The listing builds one solid part. Answer for the finished solid, in the listing's coordinates (mm). Give positions to 0.01 mm unless a question says otherwise; leave off trailing zeros. Loops run counter-clockwise (first coordinate to the right, second up) from the corner with the lowest first, then second, coordinate; pieces in that order, holes last. Notation, with made-up numbers: M 24,35.5 L 29,35.5 A32 ccw 29,68.5 Z; hole C -24,45.5 d10. An arc over 180 degrees is marked long. Use one line per item in the form item = value. Start each with the question number.
1. The part is cut by section A-A (z = 0). Write down the section's boundary in (x, y) (3 decimals), and give its area (3 significant figures).
2. The part is cut by section D-D (z = -21.5). Write down the section's boundary in (x, y), and give its area (3 significant figures).
3. The part is cut by section B-B (x = 0). Write down the section's boundary in (y, z) (3 decimals), and give its area (3 significant figures).
4. The part is cut by section C-C (y = 42). Give the number of separate pieces and of enclosed holes in the cut face, and give its area (3 significant figures).
5. Each of these flat-tipped pins is pushed along its axis until it touches: pin 1 Ø1 at (x, y) = (24.5, 52.5) entering from +Z; pin 2 Ø6 at (y, z) = (83, -5) entering from -X; pin 3 Ø5 at (x, z) = (-12.5, -25) entering from +Y; pin 4 Ø1 at (x, y) = (25.5, 52) entering from +Z. Where does it stop, or does it pass through?
6. Straight lines are drawn through the part: line 1 (X direction, y = 30, z = 0) (3 decimals); line 2 (Z direction, x = -5.5, y = 42); line 3 (Z direction, x = -16, y = 69.5). For each, find the intervals that lie inside material, in ascending order. Write a range as from..to.
7. The mould has two halves that part along Z. Classify faces 1 (the face through (-13.5, 49.3, 24.7)), 2 (the face through (9.52, 49.3, 30.22)), 3 (the face through (-14, 0, -7)): released by +Z, released by -Z, zero draft, split by the parting line, or undercut.
from build123d import *

# Parameters (mm, degrees)
SKETCH1_R           = 31.685
SKETCH1_R_2         = 14.5
BOSS_EXTRUDE1_DEPTH = 100


with BuildPart() as part:
    # Sketch1 → Boss-Extrude1 (new body)
    with BuildSketch(Plane(origin=(0, 0, 0), x_dir=(1, 0, 0), z_dir=(0, 1, 0))):
        with Locations(Location((0, 0, 0), (0, 0, 270))):
            Circle(SKETCH1_R)
        with Locations(Location((0, 0, 0), (0, 0, 270))):
            Circle(SKETCH1_R_2, mode=Mode.SUBTRACT)
        with BuildLine():
            Line((23.575325811, 10.288743262), (16.660611418, 8.042016362))
            ThreePointArc((16.660611418, 8.042016362), (10.874027167, 14.966814396), (2.5, 18.33030278))
            Line((2.5, 18.33030278), (2.5, 25.600863755))
            ThreePointArc((2.5, 25.600863755), (3.614581646, 27.93435848), (6.130131755, 28.53393961))
            ThreePointArc((6.130131755, 28.53393961), (17.154512588, 23.611160981), (25.243074312, 14.647574007))
            ThreePointArc((25.243074312, 14.647574007), (25.450186505, 12.069862926), (23.575325811, 10.288743262))
        make_face(mode=Mode.SUBTRACT)
        with BuildLine():
            Line((-2.5, 25.600863755), (-2.5, 18.33030278))
            ThreePointArc((-2.5, 18.33030278), (-10.874027167, 14.966814396), (-16.660611418, 8.042016362))
            Line((-16.660611418, 8.042016362), (-23.575325811, 10.288743262))
            ThreePointArc((-23.575325811, 10.288743262), (-25.450186505, 12.069862926), (-25.243074312, 14.647574007))
            ThreePointArc((-25.243074312, 14.647574007), (-17.154512588, 23.611160981), (-6.130131755, 28.53393961))
            ThreePointArc((-6.130131755, 28.53393961), (-3.614581646, 27.93435848), (-2.5, 25.600863755))
        make_face(mode=Mode.SUBTRACT)
        with BuildLine():
            Line((25.120410783, 5.53346068), (18.20569639, 3.28673378))
            ThreePointArc((18.20569639, 3.28673378), (17.594545551, -5.716814396), (12.79682413, -13.36006333))
            Line((12.79682413, -13.36006333), (17.070352647, -19.242070718))
            ThreePointArc((17.070352647, -19.242070718), (19.343661926, -20.474772952), (21.73120966, -19.481241021))
            ThreePointArc((21.73120966, -19.481241021), (27.756584428, -9.018660981), (29.031704092, 2.987370505))
            ThreePointArc((29.031704092, 2.987370505), (27.684120817, 5.194520069), (25.120410783, 5.53346068))
        make_face(mode=Mode.SUBTRACT)
        with BuildLine():
            Line((13.025267675, -22.180996979), (8.751739158, -16.298989592))
            ThreePointArc((8.751739158, -16.298989592), (0, -18.5), (-8.751739158, -16.298989592))
            Line((-8.751739158, -16.298989592), (-13.025267675, -22.180996979))
            ThreePointArc((-13.025267675, -22.180996979), (-13.495145967, -24.723968522), (-11.812448125, -26.687643101))
            ThreePointArc((-11.812448125, -26.687643101), (0, -29.185), (11.812448125, -26.687643101))
            ThreePointArc((11.812448125, -26.687643101), (13.495145967, -24.723968522), (13.025267675, -22.180996979))
        make_face(mode=Mode.SUBTRACT)
        with BuildLine():
            Line((-17.070352647, -19.242070718), (-12.79682413, -13.36006333))
            ThreePointArc((-12.79682413, -13.36006333), (-17.594545551, -5.716814396), (-18.20569639, 3.28673378))
            Line((-18.20569639, 3.28673378), (-25.120410783, 5.53346068))
            ThreePointArc((-25.120410783, 5.53346068), (-27.684120817, 5.194520069), (-29.031704092, 2.987370505))
            ThreePointArc((-29.031704092, 2.987370505), (-27.756584428, -9.018660981), (-21.73120966, -19.481241021))
            ThreePointArc((-21.73120966, -19.481241021), (-19.343661926, -20.474772952), (-17.070352647, -19.242070718))
        make_face(mode=Mode.SUBTRACT)
    extrude(amount=BOSS_EXTRUDE1_DEPTH)


solid = part.part
Derived:
q1.outline = M -31.685,0 L -29.185,0 L -29.185,100 L -31.685,100 Z; M -18.5,0 L -14.5,0 L -14.5,100 L -18.5,100 Z; M 14.5,0 L 18.5,0 L 18.5,100 L 14.5,100 Z; M 29.185,0 L 31.685,0 L 31.685,100 L 29.185,100 Z
q1.area = 1,300 mm2
q2.outline = M -23.27,0 L -19.74,0 L -19.74,100 L -23.27,100 Z; M -2.5,0 L 2.5,0 L 2.5,100 L -2.5,100 Z; M 19.74,0 L 23.27,0 L 23.27,100 L 19.74,100 Z
q2.area = 1,210 mm2
q3.outline = M 0,-31.685 L 100,-31.685 L 100,-14.5 L 0,-14.5 Z; M 0,14.5 L 100,14.5 L 100,18.5 L 0,18.5 Z; M 0,29.185 L 100,29.185 L 100,31.685 L 0,31.685 Z
q3.area = 2,370 mm2
q4.separate_pieces = 1
q4.enclosed_holes = 6
q4.area = 1,190 mm2
q5.pin_1 = 20.69
q5.pin_2 = -31.62
q5.pin_3 = 100
q5.pin_4 = 19.47
q6.line_1 = -31.685..-29.185, -18.5..-14.5, 14.5..18.5, 29.185..31.685
q6.line_2 = -31.2..-28.6, -17.66..-13.42, 13.42..17.66, 28.66..31.2
q6.line_3 = -27.35..-24.41, -9.29..9.29, 17.77..27.35
q7.face_1 = undercut
q7.face_2 = split by the parting line
q7.face_3 = zero draft
